Geometry: see drawing. Coordinates: mm, zero at the bounding-box minimum. Give positions to 0.01 mm unless a question says otherwise; leave off trailing zeros. Order: outer loops, then holes, each group sorted by start corner. A loop starts at its lowest first (then second) coordinate and runs counter-clockwise, first axis right, second up. Notation, with made-up numbers: M 5.25,9 L 17.25,9 A15 ccw 17.25,37 Z; hole C 68.5,3 d11. An arc over 180 degrees is marked long. Return JSON: item names as keys, results as strings.
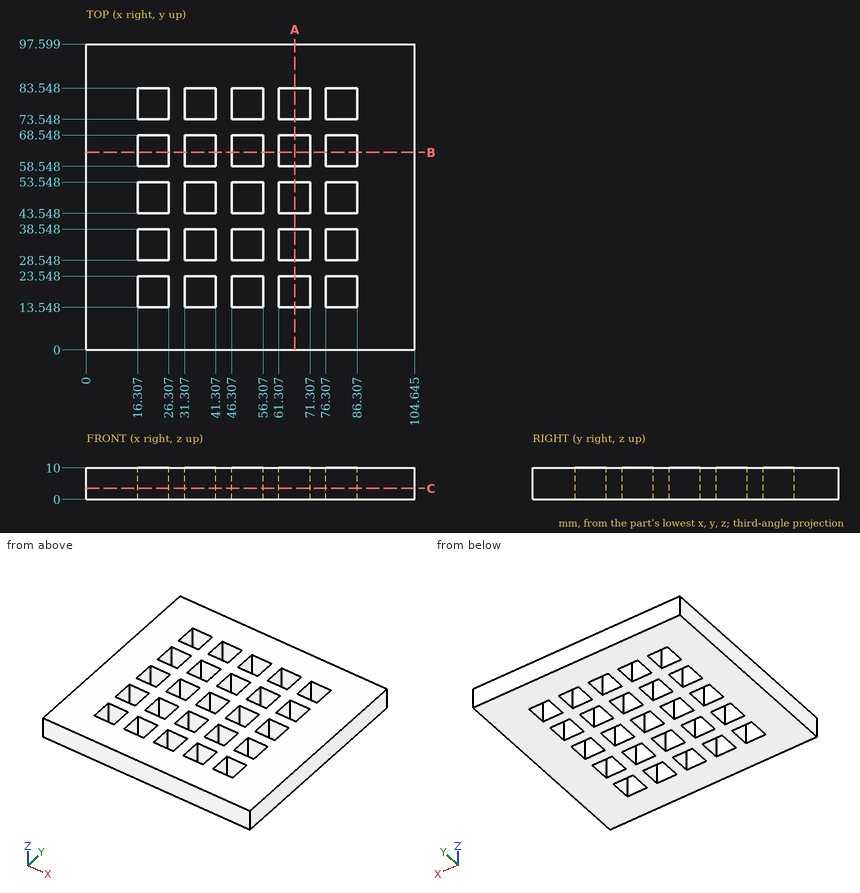
1. First-contact query: pin 1 (5 mm diameter, centred on y = 48.5, z = 2.5, fed in from -X). Flat tip, straight axial feed; report the tip coordinate or a pass-through.
Evaluation:
{"pin 1": "stops at x = 0"}
2. Section query C-C (z = 3.5). State how many separate pieces and enclosed holes the cut face has, then the cut area to 3 significant figures.
Evaluation:
{"separate pieces": "1", "enclosed holes": "25", "area": "7,710 mm^2"}
3. Section query B-B (y = 63). Return loops of the section in (x, z) (1 decimal).
Evaluation:
{"outline": "M 0,0 L 16.3,0 L 16.3,10 L 0,10 Z; M 26.3,0 L 31.3,0 L 31.3,10 L 26.3,10 Z; M 41.3,0 L 46.3,0 L 46.3,10 L 41.3,10 Z; M 56.3,0 L 61.3,0 L 61.3,10 L 56.3,10 Z; M 71.3,0 L 76.3,0 L 76.3,10 L 71.3,10 Z; M 86.3,0 L 104.6,0 L 104.6,10 L 86.3,10 Z"}
4. Section query A-A (x = 66.5). Return loops of the section in (y, z), then the cut area to 3 significant figures.
Evaluation:
{"outline": "M 0,0 L 13.55,0 L 13.55,10 L 0,10 Z; M 23.55,0 L 28.55,0 L 28.55,10 L 23.55,10 Z; M 38.55,0 L 43.55,0 L 43.55,10 L 38.55,10 Z; M 53.55,0 L 58.55,0 L 58.55,10 L 53.55,10 Z; M 68.55,0 L 73.55,0 L 73.55,10 L 68.55,10 Z; M 83.55,0 L 97.6,0 L 97.6,10 L 83.55,10 Z", "area": "476 mm^2"}
5. Ray query, probe 1 along X at (y, z) = (53.5, 8) (1 decimal); probe 2 along Y at (x, z) = (50, 6.5). Return the intervals inside material, ascending.
Evaluation:
{"probe 1": "x = 0 to 16.3, 26.3 to 31.3, 41.3 to 46.3, 56.3 to 61.3, 71.3 to 76.3, 86.3 to 104.6", "probe 2": "y = 0 to 13.55, 23.55 to 28.55, 38.55 to 43.55, 53.55 to 58.55, 68.55 to 73.55, 83.55 to 97.6"}
